from build123d import *

# Parameters (mm, degrees)
SPUR_START              = -122.221816322
SPUR_GEAR_ISO_OUTLINE_R = 1
SPUR_GEAR_ISO_DEPTH     = 3
SKETCH1_R               = 2.275
CUT_EXTRUDE1_DEPTH      = 10


# Read off the part's stored shape, not the designer's step: spur gear_iso
with BuildPart() as part:
    # spur gear_iso outline → spur gear_iso (new body)
    with BuildSketch(Plane.YZ.offset(SPUR_START)):
        with BuildLine():
            ThreePointArc((2.854590328, 8.779377764), (2.629866412, 8.827067524), (2.403998504, 8.869006051))
            ThreePointArc((2.403998504, 8.869006051), (1.695929768, 7.895188691), (1.397846451, 6.728643397))
            ThreePointArc((1.397846451, 6.728643397), (0.874053513, 6.749), (0.350260576, 6.728643397))
            ThreePointArc((0.350260576, 6.728643397), (0.052177259, 7.895188691), (-0.655891477, 8.869006051))
            ThreePointArc((-0.655891477, 8.869006051), (-0.881759385, 8.827067524), (-1.106483301, 8.779377764))
            ThreePointArc((-1.106483301, 8.779377764), (-1.387989744, 7.608721662), (-1.216965263, 6.416902795))
            ThreePointArc((-1.216965263, 6.416902795), (-1.708676972, 6.235262965), (-2.184808411, 6.016009037))
            ThreePointArc((-2.184808411, 6.016009037), (-2.906619044, 6.97968481), (-3.933453026, 7.608408563))
            ThreePointArc((-3.933453026, 7.608408563), (-4.126078584, 7.483226511), (-4.315446329, 7.353168799))
            ThreePointArc((-4.315446329, 7.353168799), (-4.127533675, 6.163895735), (-3.513438322, 5.128246912))
            ThreePointArc((-3.513438322, 5.128246912), (-3.898210152, 4.772263666), (-4.254193398, 4.387491836))
            ThreePointArc((-4.254193398, 4.387491836), (-5.289842221, 5.001587189), (-6.479115285, 5.189499843))
            ThreePointArc((-6.479115285, 5.189499843), (-6.609172997, 5.000132097), (-6.73435505, 4.80750654))
            ThreePointArc((-6.73435505, 4.80750654), (-6.105631296, 3.780672557), (-5.141955523, 3.058861924))
            ThreePointArc((-5.141955523, 3.058861924), (-5.361209451, 2.582730485), (-5.542849281, 2.091018776))
            ThreePointArc((-5.542849281, 2.091018776), (-6.734668149, 2.262043257), (-7.905324251, 1.980536814))
            ThreePointArc((-7.905324251, 1.980536814), (-7.95301401, 1.755812898), (-7.994952537, 1.529944991))
            ThreePointArc((-7.994952537, 1.529944991), (-7.021135177, 0.821876255), (-5.854589883, 0.523792937))
            ThreePointArc((-5.854589883, 0.523792937), (-5.874946486, 0), (-5.854589883, -0.523792937))
            ThreePointArc((-5.854589883, -0.523792937), (-7.021135177, -0.821876255), (-7.994952537, -1.529944991))
            ThreePointArc((-7.994952537, -1.529944991), (-7.95301401, -1.755812898), (-7.905324251, -1.980536814))
            ThreePointArc((-7.905324251, -1.980536814), (-6.734668149, -2.262043257), (-5.542849281, -2.091018776))
            ThreePointArc((-5.542849281, -2.091018776), (-5.361209451, -2.582730485), (-5.141955523, -3.058861924))
            ThreePointArc((-5.141955523, -3.058861924), (-6.105631296, -3.780672557), (-6.73435505, -4.80750654))
            ThreePointArc((-6.73435505, -4.80750654), (-6.609172997, -5.000132097), (-6.479115285, -5.189499843))
            ThreePointArc((-6.479115285, -5.189499843), (-5.289842221, -5.001587189), (-4.254193398, -4.387491836))
            ThreePointArc((-4.254193398, -4.387491836), (-3.898210153, -4.772263667), (-3.513438322, -5.128246912))
            ThreePointArc((-3.513438322, -5.128246912), (-4.127533675, -6.163895735), (-4.315446329, -7.353168799))
            ThreePointArc((-4.315446329, -7.353168799), (-4.126078584, -7.483226511), (-3.933453026, -7.608408563))
            ThreePointArc((-3.933453026, -7.608408563), (-2.906619044, -6.97968481), (-2.184808411, -6.016009037))
            ThreePointArc((-2.184808411, -6.016009037), (-1.708676972, -6.235262965), (-1.216965263, -6.416902795))
            ThreePointArc((-1.216965263, -6.416902795), (-1.387989744, -7.608721662), (-1.106483301, -8.779377764))
            ThreePointArc((-1.106483301, -8.779377764), (-0.881759385, -8.827067524), (-0.655891477, -8.869006051))
            ThreePointArc((-0.655891477, -8.869006051), (0.052177259, -7.895188691), (0.350260576, -6.728643397))
            ThreePointArc((0.350260576, -6.728643397), (0.874053513, -6.749), (1.397846451, -6.728643397))
            ThreePointArc((1.397846451, -6.728643397), (1.695929768, -7.895188691), (2.403998504, -8.869006051))
            ThreePointArc((2.403998504, -8.869006051), (2.629866412, -8.827067524), (2.854590328, -8.779377764))
            ThreePointArc((2.854590328, -8.779377764), (3.136096771, -7.608721662), (2.96507229, -6.416902795))
            ThreePointArc((2.96507229, -6.416902795), (3.456783999, -6.235262965), (3.932915438, -6.016009037))
            ThreePointArc((3.932915438, -6.016009037), (4.654726071, -6.97968481), (5.681560054, -7.608408563))
            ThreePointArc((5.681560054, -7.608408563), (5.874185611, -7.483226511), (6.063553357, -7.353168799))
            ThreePointArc((6.063553357, -7.353168799), (5.875640702, -6.163895735), (5.26154535, -5.128246912))
            ThreePointArc((5.26154535, -5.128246912), (5.64631718, -4.772263666), (6.002300425, -4.387491836))
            ThreePointArc((6.002300425, -4.387491836), (7.037949248, -5.001587189), (8.227222312, -5.189499843))
            ThreePointArc((8.227222312, -5.189499843), (8.357280024, -5.000132097), (8.482462077, -4.80750654))
            ThreePointArc((8.482462077, -4.80750654), (7.853738324, -3.780672557), (6.89006255, -3.058861924))
            ThreePointArc((6.89006255, -3.058861924), (7.109316479, -2.582730485), (7.290956308, -2.091018776))
            ThreePointArc((7.290956308, -2.091018776), (8.482775176, -2.262043257), (9.653431278, -1.980536814))
            ThreePointArc((9.653431278, -1.980536814), (9.701121037, -1.755812898), (9.743059564, -1.529944991))
            ThreePointArc((9.743059564, -1.529944991), (8.769242204, -0.821876255), (7.60269691, -0.523792937))
            ThreePointArc((7.60269691, -0.523792937), (7.623053514, 0), (7.60269691, 0.523792937))
            ThreePointArc((7.60269691, 0.523792937), (8.769242204, 0.821876255), (9.743059564, 1.529944991))
            ThreePointArc((9.743059564, 1.529944991), (9.701121037, 1.755812898), (9.653431278, 1.980536814))
            ThreePointArc((9.653431278, 1.980536814), (8.482775176, 2.262043257), (7.290956308, 2.091018776))
            ThreePointArc((7.290956308, 2.091018776), (7.109316479, 2.582730485), (6.89006255, 3.058861924))
            ThreePointArc((6.89006255, 3.058861924), (7.853738324, 3.780672557), (8.482462077, 4.80750654))
            ThreePointArc((8.482462077, 4.80750654), (8.357280024, 5.000132097), (8.227222312, 5.189499843))
            ThreePointArc((8.227222312, 5.189499843), (7.037949248, 5.001587189), (6.002300425, 4.387491836))
            ThreePointArc((6.002300425, 4.387491836), (5.64631718, 4.772263666), (5.26154535, 5.128246912))
            ThreePointArc((5.26154535, 5.128246912), (5.875640702, 6.163895735), (6.063553357, 7.353168799))
            ThreePointArc((6.063553357, 7.353168799), (5.874185611, 7.483226511), (5.681560054, 7.608408563))
            ThreePointArc((5.681560054, 7.608408563), (4.654726071, 6.97968481), (3.932915438, 6.016009037))
            ThreePointArc((3.932915438, 6.016009037), (3.456783999, 6.235262965), (2.96507229, 6.416902795))
            ThreePointArc((2.96507229, 6.416902795), (3.136096771, 7.608721662), (2.854590328, 8.779377764))
        make_face()
        with Locations((0.874053514, 0)):
            Circle(SPUR_GEAR_ISO_OUTLINE_R, mode=Mode.SUBTRACT)
    extrude(amount=SPUR_GEAR_ISO_DEPTH)

    # Sketch1 → Cut-Extrude1 (cut)
    with BuildSketch(Plane(origin=(-119.221816322, 0, 0), x_dir=(0, 0, -1), z_dir=(1, 0, 0))):
        with Locations((0, 0.874053514)):
            Circle(SKETCH1_R)
    extrude(amount=-CUT_EXTRUDE1_DEPTH, mode=Mode.SUBTRACT)


solid = part.part
CAD build for the part. Positions are in the model's coordinates, mm. A direction names the side the tool comes from. Round coordinates to 2 decimals unless told otherwise and drop trailing zeros. Order: outer loops, then holes, each group sorted by start corner. A loop starts at its lowest first (then second) coordinate and runs counter-clockwise, first axis right, second up. Notation, with made-up numbers: M -20.5,40 L 36.5,40 A18 cw 36.5,71 Z; hole C -31.5,-2.5 d3. An arc over 180 degrees is marked long. Use one line per item in the form item = value.
Q1. Saw through at A-A on z = 0. Give the cut face in (x, y), then the cut area to 3 significant figures.
Recorded:
outline = M -122.22,-5.87 L -119.22,-5.87 L -119.22,-1.4 L -122.22,-1.4 Z; M -122.22,3.15 L -119.22,3.15 L -119.22,7.62 L -122.22,7.62 Z
area = 26.8 mm^2
Q2. Which spindle directions (+Z, -Z, +X, -X, +Y, -Y) get a long thin tool onto all of the face, cutting with end or side? Do faces 5 (the cylindrical face through (-120.74, 0.88, 6.75)), 6 (the cylindrical face through (-120.7, 7.1, 2.6)), 7 (the cylindrical face through (-120.743, 4.642, -6.968)), 8 (the cylindrical face through (-120.743, -6.117, 3.793)). Say none if no direction does.
Recorded:
face_5 = +Z, +X, -X
face_6 = +X, -X
face_7 = -Z, +X, -X
face_8 = +X, -X, -Y
Q3. Saw through at B-B on z = 7. Give the cut face in (x, y).
Recorded:
outline = M -122.22,-4.31 L -119.22,-4.31 L -119.22,-2.93 L -122.22,-2.93 Z; M -122.22,-1.36 L -119.22,-1.36 L -119.22,0.32 L -122.22,0.32 Z; M -122.22,1.43 L -119.22,1.43 L -119.22,3.11 L -122.22,3.11 Z; M -122.22,4.68 L -119.22,4.68 L -119.22,6.06 L -122.22,6.06 Z
Q4. Saw through at C-C on y = -3.25. Give the cut face in (x, z).
Recorded:
outline = M -122.22,-7.25 L -119.22,-7.25 L -119.22,7.25 L -122.22,7.25 Z
Q5. Probe L1, parallel to Z at x = -120.55, y = -5.75; L2, parallel to Y at x = -119.7, z = 6.5; L3, parallel to Y at x = -121.75, z = 7.75. List the from-to ranges inside material, lowest first.
Recorded:
L1 = -5.13 to -3.45, -2.15 to 2.15, 3.45 to 5.13
L2 = -4.23 to -2.48, -1.24 to 2.99, 4.22 to 5.98
L3 = -1.38 to 0.12, 1.63 to 3.13
Q6. Two-plate mould, pull along Y, no slides. Class faces 1 (the cylindrical face through (-120.743, 8.785, -0.829)), 2 (the cylindrical face through (-120.743, -5.875, 0.007)), 3 (the cylindrical face through (-120.74, 0.87, -6.75)), 4 (the cylindrical face through (-120.74, -6.75, -2.26)): +Y half, -Y half, draft (parallel to the pull), parting line (faces both ways), or undercut.
Recorded:
face_1 = +Y half
face_2 = -Y half
face_3 = undercut
face_4 = undercut
